Autodesk Inventor part; units mm, degrees
ref_plane "YZ Plane" through (0, 0, 0) normal (1, 0, 0) x (0, 1, 0)
ref_plane "XZ Plane" through (0, 0, 0) normal (0, 1, 0) x (-1, 0, 0)
ref_plane "XY Plane" through (0, 0, 0) normal (0, 0, 1) x (1, 0, 0)
sketch "Sketch1" plane through (0, 0, 0) normal (0, 1, 0) x (-1, 0, 0)
  line L0 (0, 0) -> (220, 0)
  line L1 (220, 0) -> (220, 100)
  line L2 (220, 100) -> (0, 100)
  line L3 (0, 100) -> (0, 0)
  dimension "d11" = 220
  dimension "d16" = 100
extrude "Extrusion3" add sketch "Sketch1" along normal blind 6
sketch "Sketch3" plane through (0, 0, 0) normal (0, -1, 0) x (1, 0, 0)
  line L0 (0, 100) -> (0, 0)
  line L1 (-220, 0) -> (-220, 100)
  line L2 (-220, 85) -> (-224, 85)
  line L3 (-226, 83) -> (-226, 79)
  line L4 (-224, 77) -> (-220, 77)
  line L5 (-220, 77) -> (-220, 85)
  line L6 (-220, 54) -> (-224, 54)
  line L7 (-226, 52) -> (-226, 48)
  line L8 (-224, 46) -> (-220, 46)
  line L9 (-220, 46) -> (-220, 54)
  line L10 (-220, 23) -> (-224, 23)
  line L11 (-226, 21) -> (-226, 17)
  line L12 (-224, 15) -> (-220, 15)
  line L13 (-220, 15) -> (-220, 23)
  line L14 (0, 85) -> (4, 85)
  line L15 (6, 83) -> (6, 79)
  line L16 (4, 77) -> (0, 77)
  line L17 (0, 77) -> (0, 85)
  line L18 (0, 54) -> (4, 54)
  line L19 (6, 52) -> (6, 48)
  line L20 (4, 46) -> (0, 46)
  line L21 (0, 46) -> (0, 54)
  line L22 (0, 23) -> (4, 23)
  line L23 (6, 21) -> (6, 17)
  line L24 (4, 15) -> (0, 15)
  line L25 (0, 15) -> (0, 23)
  arc A0 (-224, 85) -> (-226, 83) centre (-224, 83) ccw
  arc A1 (-226, 79) -> (-224, 77) centre (-224, 79) ccw
  arc A2 (-224, 54) -> (-226, 52) centre (-224, 52) ccw
  arc A3 (-226, 48) -> (-224, 46) centre (-224, 48) ccw
  arc A4 (-224, 23) -> (-226, 21) centre (-224, 21) ccw
  arc A5 (-226, 17) -> (-224, 15) centre (-224, 17) ccw
  arc A6 (6, 83) -> (4, 85) centre (4, 83) ccw
  arc A7 (4, 77) -> (6, 79) centre (4, 79) ccw
  arc A8 (6, 52) -> (4, 54) centre (4, 52) ccw
  arc A9 (4, 46) -> (6, 48) centre (4, 48) ccw
  arc A10 (6, 21) -> (4, 23) centre (4, 21) ccw
  arc A11 (4, 15) -> (6, 17) centre (4, 17) ccw
  line L26 (-222, 77) -> (-222, 54) construction
  line L27 (-222, 23) -> (-222, 46) construction
  point P0 (-226, 50)
  point P1 (-220, 50)
  dimension "d35" = 2
  dimension "d36" = 8
  dimension "d37" = 6
  dimension "d38" = 8
  dimension "d39" = 8
  dimension "d40" = 8
  dimension "d41" = 8
  dimension "d42" = 8
  dimension "d43" = 6
  dimension "d44" = 23
extrude "Extrusion4" add sketch "Sketch3" against normal blind 6
sketch "Sketch4" plane through (0, 0, 0) normal (0, -1, 0) x (1, 0, 0)
  line L0 (0, 0) -> (-220, 0)
  line L1 (-220, 100) -> (0, 100)
  line L2 (-220, 54) -> (-220, 77)
  line L3 (-220, 23) -> (-220, 46)
  line L4 (-203.7, 67.75) -> (-203.7, 63.25)
  line L5 (-220, 63.25) -> (-220, 67.75)
  line L6 (-215, 70.25) -> (-207.7, 70.25)
  line L7 (-207.7, 60.75) -> (-215, 60.75)
  line L8 (-220, 67.75) -> (-215, 67.75)
  line L9 (-207.7, 67.75) -> (-203.7, 67.75)
  line L10 (-203.7, 63.25) -> (-207.7, 63.25)
  line L11 (-215, 63.25) -> (-220, 63.25)
  line L12 (-215, 60.75) -> (-215, 63.25)
  line L13 (-215, 67.75) -> (-215, 70.25)
  line L14 (-207.7, 70.25) -> (-207.7, 67.75)
  line L15 (-207.7, 63.25) -> (-207.7, 60.75)
  line L16 (-203.7, 36.75) -> (-203.7, 32.25)
  line L17 (-220, 32.25) -> (-220, 36.75)
  line L18 (-215, 39.25) -> (-207.7, 39.25)
  line L19 (-207.7, 29.75) -> (-215, 29.75)
  line L20 (-220, 36.75) -> (-215, 36.75)
  line L21 (-207.7, 36.75) -> (-203.7, 36.75)
  line L22 (-203.7, 32.25) -> (-207.7, 32.25)
  line L23 (-215, 32.25) -> (-220, 32.25)
  line L24 (-215, 29.75) -> (-215, 32.25)
  line L25 (-215, 36.75) -> (-215, 39.25)
  line L26 (-207.7, 39.25) -> (-207.7, 36.75)
  line L27 (-207.7, 32.25) -> (-207.7, 29.75)
  line L28 (-110, 100) -> (-110, 0) construction
  line L29 (-16.3, 67.75) -> (-16.3, 63.25)
  line L30 (0, 63.25) -> (0, 67.75)
  line L31 (-5, 70.25) -> (-12.3, 70.25)
  line L32 (-12.3, 60.75) -> (-5, 60.75)
  line L33 (0, 67.75) -> (-5, 67.75)
  line L34 (-12.3, 67.75) -> (-16.3, 67.75)
  line L35 (-16.3, 63.25) -> (-12.3, 63.25)
  line L36 (-5, 63.25) -> (0, 63.25)
  line L37 (-5, 60.75) -> (-5, 63.25)
  line L38 (-5, 67.75) -> (-5, 70.25)
  line L39 (-12.3, 70.25) -> (-12.3, 67.75)
  line L40 (-12.3, 63.25) -> (-12.3, 60.75)
  line L41 (0, 36.75) -> (-5, 36.75)
  line L42 (-16.3, 36.75) -> (-16.3, 32.25)
  line L43 (-16.3, 32.25) -> (-12.3, 32.25)
  line L44 (-12.3, 32.25) -> (-12.3, 29.75)
  line L45 (-12.3, 39.25) -> (-12.3, 36.75)
  line L46 (-12.3, 29.75) -> (-5, 29.75)
  line L47 (-5, 29.75) -> (-5, 32.25)
  line L48 (-5, 36.75) -> (-5, 39.25)
  line L49 (-5, 39.25) -> (-12.3, 39.25)
  line L50 (-5, 32.25) -> (0, 32.25)
  line L51 (0, 32.25) -> (0, 36.75)
  line L52 (-12.3, 36.75) -> (-16.3, 36.75)
  point P0 (-220, 65.5)
  point P1 (-220, 34.5)
  point P2 (0, 65.5)
  point P3 (0, 34.5)
  dimension "d47" = 4.5
  dimension "d48" = 2.5
  dimension "d49" = 2.5
  dimension "d50" = 5
  dimension "d51" = 4
  dimension "d52" = 7.3
  dimension "d53" = 4.5
  dimension "d54" = 2.5
  dimension "d55" = 2.5
  dimension "d56" = 5
  dimension "d57" = 4
  dimension "d58" = 7.3
extrude "Extrusion5" cut sketch "Sketch4" against normal through all
equation "\"d38\" = d36"
equation "\"d39\" = d38"
equation "\"d40\" = d36"
equation "\"d41\" = d40"
equation "\"d42\" = d41"
equation "\"d43\" = d37"
equation "\"d49\" = d48"
equation "\"d55\" = d54"
properties part number "front_panel_2004_bottom"
CAD build for the part. Positions are in the model's coordinates, mm. A direction names the side the tool comes from. Round coordinates to 2 decimals unless told otherwise and drop trailing zeros. Write each loop counter-clockwise with the first axis right and the second up, starting at its lowest first coordinate (ties: lowest second). Pieces come first, ordered by that corner, then holes. Notation, with made-up numbers: (-40, 77.25) - (-4, 77.25) arc R31 cw to (-4, 112.25) - close; hole circle Ø1 at (84, 73.5). An arc over 180 degrees is marked (long way). Return JSON: item names as keys, results as strings. Group by question number.
Item 1: 3-axis set-ups, long thin cutter, end or side, ignore diameter. For faces 1 (the face through (-222, 3, 15)), 2 (the face through (-211, 3, 60.75)), 3 (the face through (-220, 3, 59)), 4 (the face through (-2, 3, 36.75)): which of +Z, -Z, +X, -X, +Y, -Y reach the whole face in a straight line?
Item 2: Band-saw the part on A-A on z = 42.5. List the corners of the cut face in (x, y).
Item 3: Flat gauge pins, fed straight in: pin 1 Ø2 at (x, y) = (2.5, 2) entering from -Z; pin 2 Ø1 at (x, y) = (-97.5, 2.5) entering from -Z; pin 3 Ø0.8 at (y, z) = (4, 31) entering from -X; pin 4 Ø2 at (x, y) = (-221.5, 3.5) entering from +Z. Where does each tip first touch, or does it go through?
Item 4: Probe probe 1 along X at (y, z) = (1.55, 61.5); probe 2 along X at (y, z) = (4.8, 9); probe 3 along X at (y, z) = (2.85, 46.5). List the from-to ranges inside material, lowest first.
Item 5: Mould opens along X. For faces 5 (the face through (-211, 3, 29.75)), 6 (the face through (-16.3, 3, 35)), 7 (the face through (-222, 3, 85)), 8 (the face through (-220, 3, 92)) say: +X half, -X half, draft (parallel to the pull), parting line (faces both ways), or undercut.
Resolved:
{
 "1": {"face 1": "-Z, -X, +Y, -Y", "face 2": "+Y, -Y", "face 3": "-X, +Y, -Y", "face 4": "+X, +Y, -Y"},
 "2": {"outline": "(-220, 0) - (0, 0) - (0, 6) - (-220, 6) - close"},
 "3": {"pin 1": "stops at z = 15", "pin 2": "stops at z = 0", "pin 3": "stops at x = -220", "pin 4": "stops at z = 85"},
 "4": {"probe 1": "x = -220 to -215, -207.7 to -12.3, -5 to 0", "probe 2": "x = -220 to 0", "probe 3": "x = -225.32 to 5.32"},
 "5": {"face 5": "undercut", "face 6": "+X half", "face 7": "draft", "face 8": "-X half"}
}
